from build123d import *

# Parameters (mm, degrees)
BOSS_EXTRUDE1_DEPTH = 20
SKETCH4_R           = 10
BOSS_EXTRUDE3_DEPTH = 10
SKETCH5_W           = 23.907996497
SKETCH5_H           = 10.22824498
CUT_EXTRUDE2_DEPTH  = 50
BOSS_EXTRUDE4_START = 5
SKETCH7_R           = 10
BOSS_EXTRUDE4_DEPTH = 5
SKETCH11_R          = 3
BOSS_EXTRUDE7_DEPTH = 1


with BuildPart() as part:
    # Sketch2 → Boss-Extrude1 (new body)
    with BuildSketch(Plane.XY):
        with BuildLine():
            Line((-70.139472481, 19.207806068), (129.860527519, 19.207806068))
            ThreePointArc((129.860527519, 19.207806068), (136.931595331, 16.27887388), (139.860527519, 9.207806068))
            ThreePointArc((139.860527519, 9.207806068), (136.931595331, 2.136738256), (129.860527519, -0.792193932))
            Line((129.860527519, -0.792193932), (-70.139472481, -0.792193932))
            ThreePointArc((-70.139472481, -0.792193932), (-77.210540292, 2.136738256), (-80.139472481, 9.207806068))
            ThreePointArc((-80.139472481, 9.207806068), (-77.210540292, 16.27887388), (-70.139472481, 19.207806068))
        make_face()
    extrude(amount=BOSS_EXTRUDE1_DEPTH)

    # Sketch4 → Boss-Extrude3 (add)
    with BuildSketch(Plane.XZ.offset(0.792193932)):
        with Locations(Location((117.087248421, 10, 0), (0, 0, 270))):
            Circle(SKETCH4_R)
    extrude(amount=BOSS_EXTRUDE3_DEPTH)

    # Sketch5 → Cut-Extrude2 (cut)
    with BuildSketch(Plane(origin=(117, 0, 0), x_dir=(0, 0, -1), z_dir=(1, 0, 0))):
        with Locations((-10.311239758, -6.104621998)):
            Rectangle(SKETCH5_W, SKETCH5_H)
    extrude(amount=CUT_EXTRUDE2_DEPTH, mode=Mode.SUBTRACT)

    # Sketch7 → Boss-Extrude4 (add)
    with BuildSketch(Plane(origin=(0, 0, 0), x_dir=(-1, 0, 0), z_dir=(0, 0, -1)).offset(BOSS_EXTRUDE4_START)):
        with Locations((70.139472481, 9.207806068)):
            Circle(SKETCH7_R)
    extrude(amount=-BOSS_EXTRUDE4_DEPTH)

    # Sketch11 → Boss-Extrude7 (add)
    with BuildSketch(Plane(origin=(117, 0, 0), x_dir=(0, 0, -1), z_dir=(1, 0, 0))):
        with Locations((-14.992294677, -7.514688693)):
            Circle(SKETCH11_R)
        with Locations((-5, -7.514688693)):
            Circle(SKETCH11_R)
    extrude(amount=BOSS_EXTRUDE7_DEPTH)


solid = part.part
Geometry check sheet. Reference: the model listing, model coordinates, mm. A direction names the side the tool comes from. Round coordinates to 2 decimals unless told otherwise and drop trailing zeros. Loops run counter-clockwise (first coordinate to the right, second up) from the corner with the lowest first, then second, coordinate; pieces in that order, holes last. Notation, with made-up numbers: (64, 43) -> (102, 43) arc R10 ccw to (102, 62) -> close; hole circle Ø5 at (-40, 26.5). An arc over 180 degrees is marked (long way). Answer as a JSON object with one key per item and string values. Group by question number.
Item 1: Cross-section at A-A, the plane z = 5. Record the cut outline in (x, y), plus the area to 3 significant figures.
Item 2: Cross-section at B-B, the plane x = 94.5. Record the cut outline in (y, z), plus the area to 3 significant figures.
Item 3: Cross-section at C-C, the plane y = 4. Record the cut outline in (x, z).
Item 4: Release check for a two-part mould opening along Y. For faces 5 (the face through (25, -0.792, 10)), 6 (the face through (118, -7, 5)), 7 (the face through (117.493, -9.34, 17.373)) record: pulls with the +Y half, pulls with the -Y half, needs draft (parallel to the pull), parting line crosses it, or undercut.
Item 5: Depth check by flat-ended pin: pin 1 Ø1 at (x, z) = (-1.5, 7.5) entering from -Y; pin 2 Ø4 at (x, z) = (124, 7.5) entering from -Y; pin 3 Ø6 at (x, y) = (22.5, 12.5) entering from -Z. Enter the tip coordinate at first touch or a pass-through.
Item 6: Cross-section at D-D, the plane y = 13.5. Record the cut outline in (x, z), plus the area to 3 significant figures.
Item 7: Set-up check for faces 1 (the face through (128, -0.792, 10)), 2 (the face through (118, -7, 15)), 3 (the face through (28, 19.208, 10)), 4 (the face through (117.49, -10.18, 3.62)): record each of +Z, -Z, +X, -X, +Y, -Y from which the full face is reachable in a straight line by a thin tool's end or side.
Item 8: Thickness scan on line 1 along Z through (x, y) = (-53.5, 9.5); line 2 along Y through (x, z) = (-39.5, 15); line 3 along X through (y, z) = (8.5, 14.5). Record the ranges inside material, lowest first.
Determined:
{
 "1": {"outline": "(-70.14, -0.79) -> (108.43, -0.79) -> (108.43, -10.79) -> (117, -10.79) -> (117, -10.51) -> (118, -10.51) -> (118, -4.51) -> (117, -4.51) -> (117, -0.99) -> (125.75, -0.99) -> (125.75, -0.79) -> (129.86, -0.79) arc R10 ccw to (129.86, 19.21) -> (-70.14, 19.21) arc R10 ccw to start", "area": "4,410 mm²"},
 "2": {"outline": "(-0.79, 0) -> (19.21, 0) -> (19.21, 20) -> (-0.79, 20) -> close", "area": "400 mm²"},
 "3": {"outline": "(-78.68, -5) -> (-61.6, -5) -> (-61.6, 0) -> (138.4, 0) -> (138.4, 20) -> (-78.68, 20) -> close"},
 "4": {"face 5": "pulls with the -Y half", "face 6": "needs draft", "face 7": "undercut"},
 "5": {"pin 1": "stops at y = -0.79", "pin 2": "stops at y = -0.99", "pin 3": "stops at z = 0"},
 "6": {"outline": "(-79.17, -5) -> (-61.11, -5) -> (-61.11, 0) -> (138.89, 0) -> (138.89, 20) -> (-79.17, 20) -> close", "area": "4,450 mm²"},
 "7": {"face 1": "+X, -Y", "face 2": "+Z, -Z, +X, -Y", "face 3": "+Z, -Z, +X, -X, +Y", "face 4": "+X"},
 "8": {"line 1": "z = 0 to 20", "line 2": "y = -0.79 to 19.21", "line 3": "x = -80.11 to 139.84"}
}
